Part model, mm, in its own coordinate system. Give positions to 0.01 mm unless a question says otherwise; leave off trailing zeros. Write each loop counter-clockwise with the first axis right and the second up, starting at its lowest first coordinate (ties: lowest second). Pieces come first, ordered by that corner, then holes. Notation, with made-up numbers: (7, 52) - (42, 52) arc R5 ccw to (42, 58) - close; hole circle Ø7 at (12.25, 83.25). An arc over 180 degrees is marked (long way). Answer as a JSON object with one key per item and string values. Group by question number.
```python
from build123d import *

# Parameters (mm, degrees)
SKETCH1_W            = 80
SKETCH1_H            = 64
BOSS_EXTRUDE1_DEPTH  = 10
LPATTERN1_COUNT      = 3
LPATTERN1_PITCH      = 32.5
LPATTERN1_COUNT_DIR2 = 2
LPATTERN1_PITCH_DIR2 = 52


with BuildPart() as part:
    # Sketch1 → Boss-Extrude1 (new body)
    with BuildSketch(Plane.XY):
        with Locations((40, 0)):
            Rectangle(SKETCH1_W, SKETCH1_H)
    extrude(amount=BOSS_EXTRUDE1_DEPTH)

    # Sketch4 → M6 Clearance Hole1 (revolve, cut)
    with BuildSketch(Plane(origin=(7.5, -26, 10), x_dir=(0, -1, 0), z_dir=(1, 0, 0))):
        Polygon((0, 0), (0, 28.103012167), (3.5, 26), (3.5, 0), align=None)
    m6_clearance_hole1 = revolve(axis=Axis((7.5, -26, 16.35), (0, 0, -1)), mode=Mode.SUBTRACT)

    # LPattern1: M6 Clearance Hole1 3 × 2
    with Locations(*[(i * LPATTERN1_PITCH, j * LPATTERN1_PITCH_DIR2, 0) for i in range(LPATTERN1_COUNT) for j in range(LPATTERN1_COUNT_DIR2) if (i, j) != (0, 0)]):
        add(m6_clearance_hole1, mode=Mode.SUBTRACT)


solid = part.part
```
1) Band-saw the part on C-C (y = 26). List the corners of the cut face in (x, z).
2) Band-saw the part on B-B (x = 40). List the corners of the cut face in (y, z), plus the area to 3 significant figures.
3) Mould opens along X. For faces 1 (the flat face through (0, 0, 5)), 2 (the flat face through (39, 0, 0)), 3 (the cylindrical face through (75.605, 24.385, 5.07)), 4 (the flat face through (80, 0, 5)) say: pulls with the +X half, pulls with the -X half, needs draft (parallel to the pull), parting line crosses it, or undercut.
4) Band-saw the part on A-A (z = 5.25). List the corners of the cut face in (x, y).
5) Drop a flat-ended pin along its axis: P1, Ø6.5, axis at x = 72.5, y = 26, coming from the -Z side. Give the stop position or say it passes through.
6) Probe line 1 (X direction, y = 26, z = 2); line 2 (Y direction, x = 7.5, z = 5); line 3 (X direction, y = -23.5, z = 3.5). List the from-to ranges inside material, lowest first.
Verdict:
{
 "1": {"outline": "(0, 0) - (4, 0) - (4, 10) - (0, 10) - close; (11, 0) - (36.5, 0) - (36.5, 10) - (11, 10) - close; (43.5, 0) - (69, 0) - (69, 10) - (43.5, 10) - close; (76, 0) - (80, 0) - (80, 10) - (76, 10) - close"},
 "2": {"outline": "(-32, 0) - (-29.5, 0) - (-29.5, 10) - (-32, 10) - close; (-22.5, 0) - (22.5, 0) - (22.5, 10) - (-22.5, 10) - close; (29.5, 0) - (32, 0) - (32, 10) - (29.5, 10) - close", "area": "500 mm2"},
 "3": {"face 1": "pulls with the -X half", "face 2": "needs draft", "face 3": "undercut", "face 4": "pulls with the +X half"},
 "4": {"outline": "(0, -32) - (80, -32) - (80, 32) - (0, 32) - close; hole circle Ø7 at (7.5, -26); hole circle Ø7 at (7.5, 26); hole circle Ø7 at (40, -26); hole circle Ø7 at (40, 26); hole circle Ø7 at (72.5, -26); hole circle Ø7 at (72.5, 26)"},
 "5": {"P1": "through"},
 "6": {"line 1": "0 to 4, 11 to 36.5, 43.5 to 69, 76 to 80", "line 2": "-32 to -29.5, -22.5 to 22.5, 29.5 to 32", "line 3": "0 to 5.05, 9.95 to 37.55, 42.45 to 70.05, 74.95 to 80"}
}
